from build123d import *

# Parameters (mm, degrees)
BOSS_EXTRUDE1_DEPTH                             = 4
SKETCH2_R                                       = 2.5
BOSS_EXTRUDE2_DEPTH                             = 15
SKETCH3_W                                       = 51
SKETCH3_H                                       = 31
CUT_EXTRUDE1_DEPTH                              = 15
CSK_FOR_M2_FLAT_HEAD_MACHINE_SCREW1_D           = 2.4
CSK_FOR_M2_FLAT_HEAD_MACHINE_SCREW1_DEPTH       = 58
CSK_FOR_M2_FLAT_HEAD_MACHINE_SCREW1_CSINK_D     = 4.4
CSK_FOR_M2_FLAT_HEAD_MACHINE_SCREW1_CSINK_ANGLE = 90
CSK_FOR_M2_FLAT_HEAD_MACHINE_SCREW1_TIP         = 0.721032743


# Read off the part's stored shape, not the designer's step: Boss-Extrude1
with BuildPart() as part:
    # Boss-Extrude1 outline → Boss-Extrude1 (new body)
    with BuildSketch(Plane(origin=(0, 0, 0), x_dir=(1, 0, 0), z_dir=(0, 1, 0))):
        with BuildLine():
            ThreePointArc((100.769776489, 8.232980914), (105.012417176, 9.990340227), (106.769776489, 14.232980914))
            Line((106.769776489, 14.232980914), (106.769776489, 132.22554715))
            add(Edge.make_bspline(
                [(106.769776489, 132.22554715), (106.769776489, 159.234690285), (66.769776489, 155.557917259), (71.369776489, 140.524437357), (43.491097907, 140.524437357), (48.091097907, 155.557917259), (8.091097907, 159.234690285), (8.091097907, 132.236386798)],
                knots=[0, 0, 0, 0, 0, 0, 0, 0, 1, 1, 1, 1, 1, 1, 1, 1], degree=7))
            Line((8.091097907, 132.236386798), (8.091097907, 14.232980914))
            ThreePointArc((8.091097907, 14.232980914), (9.84845722, 9.990340227), (14.091097907, 8.232980914))
            Line((14.091097907, 8.232980914), (100.769776489, 8.232980914))
        make_face()
    extrude(amount=BOSS_EXTRUDE1_DEPTH)

    # Sketch2 → Boss-Extrude2 (add)
    with BuildSketch(Plane(origin=(0, 4, 0), x_dir=(1, 0, 0), z_dir=(0, 1, 0))):
        with Locations(Location((32.161972906, 83.24092865, 0), (0, 0, 270))):
            Circle(SKETCH2_R)
        with Locations(Location((82.067189883, 83.24092865, 0), (0, 0, 270))):
            Circle(SKETCH2_R)
        with Locations(Location((32.161972906, 24.49174917, 0), (0, 0, 270))):
            Circle(SKETCH2_R)
        with Locations(Location((84.053708344, 24.49174917, 0), (0, 0, 270))):
            Circle(SKETCH2_R)
    extrude(amount=BOSS_EXTRUDE2_DEPTH)

    # Sketch3 → Cut-Extrude1 (cut)
    with BuildSketch(Plane(origin=(0, 4, 0), x_dir=(1, 0, 0), z_dir=(0, 1, 0))):
        with Locations((81.269776489, 116.201924425)):
            Rectangle(SKETCH3_W, SKETCH3_H)
    extrude(amount=-CUT_EXTRUDE1_DEPTH, mode=Mode.SUBTRACT)

    # CSK for M2 Flat Head Machine Screw1
    with Locations(Plane(origin=(17.058706918, 0, -139.962329176), x_dir=(0, 0, -1), z_dir=(0, -1, 0))):
        with Locations((0, 0), (0, 79.68146648), (-120.125549754, 0), (-120.125549754, 79.68146648)):
            CounterSinkHole(CSK_FOR_M2_FLAT_HEAD_MACHINE_SCREW1_D / 2, CSK_FOR_M2_FLAT_HEAD_MACHINE_SCREW1_CSINK_D / 2, depth=CSK_FOR_M2_FLAT_HEAD_MACHINE_SCREW1_DEPTH, counter_sink_angle=CSK_FOR_M2_FLAT_HEAD_MACHINE_SCREW1_CSINK_ANGLE)
            with Locations((0, 0, -(CSK_FOR_M2_FLAT_HEAD_MACHINE_SCREW1_DEPTH + CSK_FOR_M2_FLAT_HEAD_MACHINE_SCREW1_TIP / 2))):  # 118° drill point
                Cone(0, CSK_FOR_M2_FLAT_HEAD_MACHINE_SCREW1_D / 2, CSK_FOR_M2_FLAT_HEAD_MACHINE_SCREW1_TIP, mode=Mode.SUBTRACT)


solid = part.part
CAD build for the part. Positions are in the model's coordinates, mm. A direction names the side the tool comes from. Coordinates: 2 decimals unless noted, no trailing zeros. Write each loop counter-clockwise with the first axis right and the second up, starting at its lowest first coordinate (ties: lowest second). Pieces come first, ordered by that corner, then holes. Notation, with made-up numbers: (88.25, 5.25) - (93.25, 5.25) arc R25 ccw to (93.25, 30.25) - close; hole circle Ø9 at (54, 63). An arc over 180 degrees is marked (long way). Use a Markdown table: item, result. Add a question column.
Item 1: Band-saw the part on B-B, the plane z = -94. Give the cut face in (x, y).
Item 2: Drill centre lines: L1, parallel to Z at x = 32.5, y = 12.75; L2, parallel to Y at x = 16, z = -61; L3, parallel to Z at x = 30, y = 11.25. Where is each one in solid material? Low to high. Write a range as from..to.
Item 3: Band-saw the part on A-A, the plane y = 16.5. Give the cut face in (x, z).
Item 4: Flat gauge pins, fed straight in: pin 1 (1 mm diameter, centred on x = 60, z = -77.5, fed in from +Y); pin 2 (2 mm diameter, centred on x = 96.74, z = -139.96, fed in from +Y); pin 3 (2 mm diameter, centred on x = 72.5, y = 1.5, fed in from -Z); pin 4 (3 mm diameter, centred on y = 2, z = -119.5, fed in from +X). Where does each tip first touch, or does it go through?
Item 5: 3-axis set-ups, long thin cutter, end or side, ignore diameter. For faces 1 (the face through (57, 2, -8.233)), 2 (the face through (31.204, 11.395, -80.932)), 3 (the face through (55.77, 2, -116)): which of +Z, -Z, +X, -X, +Y, -Y reach the whole face in a straight line?
Item 6: Mould opens along X. For faces 4 (the face through (32, 19, -83)), 5 (the face through (29.72, 11.4, -25.03)), 6 (the face through (79.85, 11.4, -82.09)), 7 (the face through (106.77, 2, -57)) say: pulls with the +X half, pulls with the -X half, needs draft (parallel to the pull), parting line crosses it, or undercut.
Numbers:
| question | item | result |
|---|---|---|
| 1 | outline | (8.09, 0) - (106.77, 0) - (106.77, 4) - (8.09, 4) - close |
| 2 | L1 | -85.72..-80.76, -26.97..-22.01 |
| 2 | L2 | 0..4 |
| 2 | L3 | -84.5..-81.99, -25.75..-23.24 |
| 3 | outline | circle Ø5 at (32.16, -83.24); circle Ø5 at (32.16, -24.49); circle Ø5 at (82.07, -83.24); circle Ø5 at (84.05, -24.49) |
| 4 | pin 1 | y = 4 |
| 4 | pin 2 | through |
| 4 | pin 3 | z = -149.05 |
| 4 | pin 4 | x = 55.77 |
| 5 | face 1 | +Z, +X, -X, +Y, -Y |
| 5 | face 2 | +Y |
| 5 | face 3 | +X, +Y, -Y |
| 6 | face 4 | needs draft |
| 6 | face 5 | undercut |
| 6 | face 6 | undercut |
| 6 | face 7 | pulls with the +X half |
